from build123d import *

# Parameters (mm, degrees)
EXTRUDE_1_DEPTH          = 20
SHELL_1_T                = -6
CUT_EXTRUDE_2_DEPTH      = 110.544511501
CUT_EXTRUDE_2_DEPTH_BACK = 110.544511501
SKETCH_4_R               = 8
SKETCH_4_W               = 28
SKETCH_4_H               = 48.08326112
EXTRUDE_5_DEPTH          = 6


with BuildPart() as part:
    # 草圖1 → 伸長1 (new, symmetric)
    with BuildSketch(Plane(origin=(0, 0, 0), x_dir=(1, 0, 0), z_dir=(0, 1, 0))):
        with BuildLine():
            Line((56.455835634, -20), (-48, -20))
            ThreePointArc((-48, -20), (-56.485281374, -23.514718626), (-60, -32))
            Line((-60, -32), (-100, -32))
            Line((-100, -32), (-100, 0))
            ThreePointArc((-100, 0), (-94.142135624, 14.142135624), (-80, 20))
            Line((-80, 20), (56.455835634, 20))
            Line((56.455835634, 20), (56.455835634, -20))
        make_face()
    extrude(amount=EXTRUDE_1_DEPTH, both=True)

    # 薄殼1
    shell_1_openings = [part.faces().sort_by_distance(p)[0] for p in [
        (-80, 0, 32),
        (56.455835634, 0, 0),
    ]]
    offset(amount=SHELL_1_T, openings=shell_1_openings, kind=Kind.INTERSECTION)

    # 草圖3 → 伸長2 (cut, two sides: drawn at the far end of the back side and taken through both)
    with BuildSketch(Plane.XY.offset(20).offset(-CUT_EXTRUDE_2_DEPTH_BACK)):
        Polygon((-238.812297792, 238.812297792), (-31.748125619, 31.748125619), (31.647752007, -31.647752007), (238.711924181, -238.711924181), (652.840268527, 175.416420166), (175.316046555, 652.940642138), align=None)
    extrude(amount=CUT_EXTRUDE_2_DEPTH + CUT_EXTRUDE_2_DEPTH_BACK, mode=Mode.SUBTRACT)

    # 草圖4 → 伸長5 (add)
    with BuildSketch(Plane(origin=(0, 0, 0), x_dir=(0, 0, -1), z_dir=(0.7071067811865488, 0.7071067811865464, 0))):
        with BuildLine():
            Line((32, -29.988893001), (32, 45))
            ThreePointArc((32, 45), (24, 58.856406461), (8, 58.856406461))
            Line((8, 58.856406461), (-27, 38.649147039))
            ThreePointArc((-27, 38.649147039), (-30.660254038, 34.988893001), (-32, 29.988893001))
            Line((-32, 29.988893001), (-32, -45))
            ThreePointArc((-32, -45), (-24, -58.856406461), (-8, -58.856406461))
            Line((-8, -58.856406461), (27, -38.649147039))
            ThreePointArc((27, -38.649147039), (30.660254038, -34.988893001), (32, -29.988893001))
        make_face()
        with Locations(Location((16, 45, 0), (0, 0, 90))):
            Circle(SKETCH_4_R, mode=Mode.SUBTRACT)
        with Locations(Location((-16, -45, 0), (0, 0, 90))):
            Circle(SKETCH_4_R, mode=Mode.SUBTRACT)
        with Locations((0, 4.242640687)):
            Rectangle(SKETCH_4_W, SKETCH_4_H, mode=Mode.SUBTRACT)
    extrude(amount=-EXTRUDE_5_DEPTH)


solid = part.part
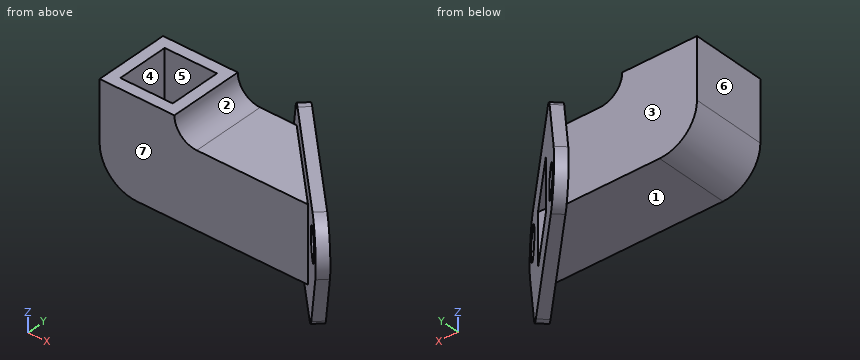
Read the model definition and answer for the solid it produces. Units are mm, in the model's axes. Face numbers are marked on the shaded views. A direction names the side the tool comes from. Coordinates: 2 decimals unless noted, no trailing zeros. Order: outer loops, then holes, each group sorted by start corner. A loop starts at its lowest first (then second) coordinate and runs counter-clockwise, first axis right, second up. Notation, with made-up numbers: M 5,83 L 46,83 A13 ccw 46,103 Z; hole C 41.5,23.25 d6. An arc over 180 degrees is marked long. Put each result on its own line as item: value. Start each with the question number.
Item 1: Consider probe 1 along Y at (x, z) = (-81, 14.5); probe 2 along X at (y, z) = (-9.5, 27.5); probe 3 along Y at (x, z) = (-38, 6). Determine where each line is inside the solid, lowest interval first. Write a range as [from, to].
Item 2: Given pin 1 Ø14 at (x, y) = (-24.5, -4.5) entering from -Z; pin 2 Ø5 at (y, z) = (-38, 25.5) entering from -X; pin 3 Ø8 at (x, z) = (25, 1.5) entering from -Y, each flat-ended and moving along its own axis, determine where each tip first touches the part or whether it passes through.
Item 3: Section A-A, the plane x = -70.5 is taken. Determine the outline of the cut face in (y, z).
Item 4: For the marked faces 1, 2 and 3, determine the directions among +Z, -Z, +X, -X, +Y, -Y from which every point of the face is accessible in a straight line to the end or side of a thin tool.
Item 5: The mould has two halves that part along Y. Classify the marked faces 4, 5, 6 and 7: +Y half, -Y half, draft (parallel to the pull), parting line (faces both ways), or undercut.
Item 6: Section D-D, the plane x = -2 is taken. Determine the outline of the cut face in (y, z).
Item 7: Section B-B, the plane y = -0.5 is taken. Determine the outline of the cut face in (x, z), plus the area to 3 significant figures.
Item 8: Section C-C, the plane x = -19.5 is taken. Determine the outline of the cut face in (y, z).
Computed:
1. probe 1: y = [-20, -14], [14, 20]
1. probe 2: x = [-100, -94], [-65.43, -59.12], [1.01, 9.5]
1. probe 3: y = [-20, -14], [14, 20], [29.51, 33.8]
2. pin 1: stops at z = -20
2. pin 2: stops at x = 27.01
2. pin 3: stops at y = -37.49
3. outline: M -20,-20 L 20,-20 L 20,32 L 14,32 L 14,-14 L -14,-14 L -14,32 L -20,32 Z
4. face 1: -Z, -X, -Y
4. face 2: +Z, +Y, -Y
4. face 3: +Z, -Z, -X
5. face 4: undercut
5. face 5: undercut
5. face 6: draft
5. face 7: -Y half
6. outline: M -20,-20 L -6.49,-20 L -6.49,-32 L 2,-32 L 2,-14 L -14,-14 L -14,14 L 2,14 L 2,32 L -6.49,32 L -6.49,20 L -20,20 Z
7. outline: M -100,0 A20 ccw -80,-20 L -7.99,-20 L -7.99,-32 L 0.5,-32 L 0.5,-14 L -80,-14 A14 cw -94,0 L -94,32 L -100,32 Z; M -66,32 A18 ccw -48,14 L 0.5,14 L 0.5,32 L -7.99,32 L -7.99,20 L -48,20 A12 cw -60,32 Z
7. area: 1,470 mm2
8. outline: M -20,-20 L 11.01,-20 L 11.01,-32 L 19.5,-32 L 19.5,32 L 11.01,32 L 11.01,20 L -20,20 Z; hole M -14,-14 L 14,-14 L 14,14 L -14,14 Z
